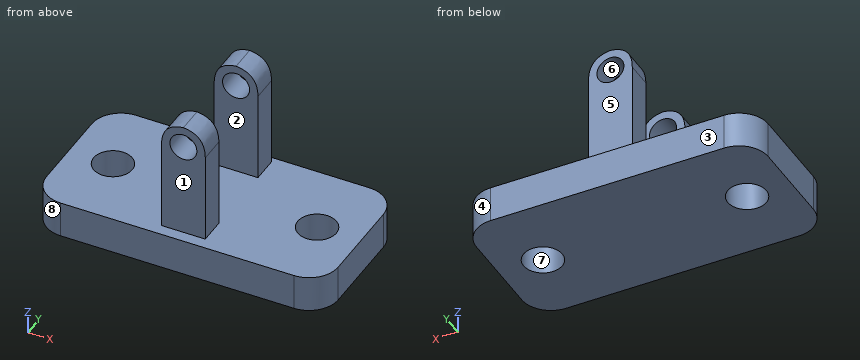
```python
from build123d import *

# Parameters (mm, degrees)
F0_W        = 50.8
F0_H        = 25.4
F0_R        = 3.3655
F1_DEPTH    = 6.35
F2_R        = 5.08
F3_W        = 7.62
F3_H        = 4.572
F4_DEPTH    = 20.32
F5_R        = 2.3495
F6_DEPTH    = 25.4
F7_T1_DEPTH = 27.432
F7_T3_DEPTH = 27.432


# Not quite as in the source:
# - a fillet or chamfer that OpenCascade refuses, or shapes differently, is made with other operations: its cross-section is extruded or revolved along the edge and cut away or added


with BuildPart() as f1:
    # F0 (on Top) → F1 (new body)
    with BuildSketch(Plane.XY):
        with Locations((14.6050021708, 1.6630402533)):
            Rectangle(F0_W, F0_H)
        with Locations((-3.1749978292, 1.6630402533)):
            Circle(F0_R, mode=Mode.SUBTRACT)
        with Locations((32.3850021708, 1.6630402533)):
            Circle(F0_R, mode=Mode.SUBTRACT)
    extrude(amount=F1_DEPTH)

    # F2
    f2_edges = [f1.edges().sort_by_distance(p)[0] for p in [
        (40.005002, -11.03696, 3.175),
        (40.005002, 14.36304, 3.175),
        (-10.794998, -11.03696, 3.175),
        (-10.794998, 14.36304, 3.175),
    ]]
    fillet(f2_edges, radius=F2_R)

    # F3 (on face) → F4 (join)
    with BuildSketch(Plane.XY.offset(6.35)):
        with Locations((14.6050021708, 11.0610402533)):
            Rectangle(F3_W, F3_H)
        with Locations((14.6050021708, -6.7189597467)):
            Rectangle(F3_W, F3_H)
    extrude(amount=F4_DEPTH)

    # F5 (on face) → F6 (cut)
    with BuildSketch(Plane(origin=(0, 13.3470402533, 0), x_dir=(-1, 0, 0), z_dir=(0, 1, 0))):
        with Locations((-14.6050021708, 22.86)):
            Circle(F5_R)
    extrude(amount=-F6_DEPTH, mode=Mode.SUBTRACT)

    # F7: fillet of radius 4.572 on 4 edges, made by hand

    # F7_s2 → F7_t1 (cut)
    with BuildSketch(Plane.XZ.offset(-6.9970402533)):
        with BuildLine():
            add(Edge.make_bspline(
                [(18.4150021708, 22.098), (18.4150021708, 26.67), (13.8430021708, 26.67)],
                knots=[0, 0, 0, 1, 1, 1], degree=2, weights=[1, 1, 1]))
            Line((13.8430021708, 26.67), (18.4150021708, 26.67))
            Line((18.4150021708, 26.67), (18.4150021708, 22.098))
        make_face()
        with BuildLine():
            add(Edge.make_bspline(
                [(10.7950021708, 22.098), (10.7950021708, 26.67), (15.3670021708, 26.67)],
                knots=[0, 0, 0, 1, 1, 1], degree=2, weights=[1, 1, 1]))
            Line((15.3670021708, 26.67), (10.7950021708, 26.67))
            Line((10.7950021708, 26.67), (10.7950021708, 22.098))
        make_face()
    extrude(amount=F7_T1_DEPTH, mode=Mode.SUBTRACT)

    # F7_s4 → F7_t3 (cut)
    with BuildSketch(Plane.XZ.offset(-24.7770402533)):
        with BuildLine():
            add(Edge.make_bspline(
                [(18.4150021708, 22.098), (18.4150021708, 26.67), (13.8430021708, 26.67)],
                knots=[0, 0, 0, 1, 1, 1], degree=2, weights=[1, 1, 1]))
            Line((13.8430021708, 26.67), (18.4150021708, 26.67))
            Line((18.4150021708, 26.67), (18.4150021708, 22.098))
        make_face()
        with BuildLine():
            add(Edge.make_bspline(
                [(10.7950021708, 22.098), (10.7950021708, 26.67), (15.3670021708, 26.67)],
                knots=[0, 0, 0, 1, 1, 1], degree=2, weights=[1, 1, 1]))
            Line((15.3670021708, 26.67), (10.7950021708, 26.67))
            Line((10.7950021708, 26.67), (10.7950021708, 22.098))
        make_face()
    extrude(amount=F7_T3_DEPTH, mode=Mode.SUBTRACT)


solid = f1.part
```
Verification items for the finished model (mm, model axes). Face numbers are marked on the shaded views. A direction names the side the tool comes from. Coordinates: 2 decimals unless noted, no trailing zeros. Order: outer loops, then holes, each group sorted by start corner. A loop starts at its lowest first (then second) coordinate and runs counter-clockwise, first axis right, second up. Notation, with made-up numbers: (69, 78) -> (102, 78) arc R38 ccw to (102, 116) -> close; hole circle Ø1 at (31, 26.5). An arc over 180 degrees is marked (long way). Answer as CSV lines item,"result". Start each with the question number.
1) Gauge pin test, flat ends, axial feed: pin 1 Ø2.5 at (y, z) = (10, 16.5) entering from +X (3 decimals); pin 2 Ø3 at (x, z) = (14.61, 22.86) entering from -Y; pin 3 Ø1.5 at (x, y) = (33, -6.5) entering from +Z; pin 4 Ø6 at (x, z) = (15, 19.5) entering from -Y. Record the tip position at first contact, or that the pin passes through.
2) Set-up check for the marked faces 1, 2, 3, 4 and 5: record each of +Z, -Z, +X, -X, +Y, -Y from which the full face is reachable in a straight line by a thin tool's end or side.
3) Material ranges on L1, parallel to Y at x = 15, z = 13.25; L2, parallel to X at y = 4, z = 3.75 (3 decimals); L3, parallel to Z at x = 1.5, y = -9, recorded low to high. Write a range as [from, to].
4) Cross-section at A-A, the plane z = 17.5. Record the boundary of the cut face in (x, y) (3 decimals).
5) Cross-section at C-C, the plane z = 3.5. Record the boundary of the cut face in (x, y) (1 decimal).
6) Cross-section at B-B, the plane y = 8. Record the boundary of the cut face in (x, z) (3 decimals), then the cut area to 3 significant figures.
7) Release check for a two-part mould opening along Y. For the marked faces 6, 7 and 8 record: released by +Y, released by -Y, zero draft, split by the parting line, or undercut.
8) Cross-section at D-D, the plane x = 9. Record the boundary of the cut face in (y, z), then the cut area to 3 significant figures.
Conclusion:
1,pin 1,"stops at x = 18.415"
1,pin 2,"passes through"
1,pin 3,"stops at z = 6.35"
1,pin 4,"stops at y = -9"
2,face 1,"+Z, +X, -X, -Y"
2,face 2,"+Z, +X, -X"
2,face 3,"+Z, -Z, +X, -X, +Y"
2,face 4,"+Z, -Z, +X, +Y"
2,face 5,"+Z, +X, -X, +Y"
3,L1,"y = [-9, -4.43], [8.78, 13.35]"
3,L2,"x = [-10.795, -5.597], [-0.753, 29.963], [34.807, 40.005]"
3,L3,"z = [0, 6.35]"
4,outline,"(10.795, -9.005) -> (18.415, -9.005) -> (18.415, -4.433) -> (10.795, -4.433) -> close; (10.795, 8.775) -> (18.415, 8.775) -> (18.415, 13.347) -> (10.795, 13.347) -> close"
5,outline,"(-10.8, -6) arc R5.1 ccw to (-5.7, -11) -> (34.9, -11) arc R5.1 ccw to (40, -6) -> (40, 9.3) arc R5.1 ccw to (34.9, 14.4) -> (-5.7, 14.4) arc R5.1 ccw to (-10.8, 9.3) -> close; hole circle Ø6.7 at (-3.2, 1.7); hole circle Ø6.7 at (32.4, 1.7)"
6,outline,"(-10.795, 0) -> (40.005, 0) -> (40.005, 6.35) -> (-10.795, 6.35) -> close"
6,area,"323 mm²"
7,face 6,"zero draft"
7,face 7,"undercut"
7,face 8,"released by -Y"
8,outline,"(-11.04, 0) -> (14.36, 0) -> (14.36, 6.35) -> (-11.04, 6.35) -> close"
8,area,"161 mm²"
